For this review, use the dimensioned drawing (mm, ordinates from the lowest corner) and the shaded views. A direction names the side the tool comes from. Coordinates: 2 decimals unless noted, no trailing zeros. Write each loop counter-clockwise with the first axis right and the second up, starting at its lowest first coordinate (ties: lowest second). Pieces come first, ordered by that corner, then holes. Notation, with made-up numbers: M 27.25,49.25 L 69.25,49.25 A12 ccw 69.25,63.25 Z; hole C 1.25,35 d8. An arc over 180 degrees is marked long. One line per question, with ' | ' between items.
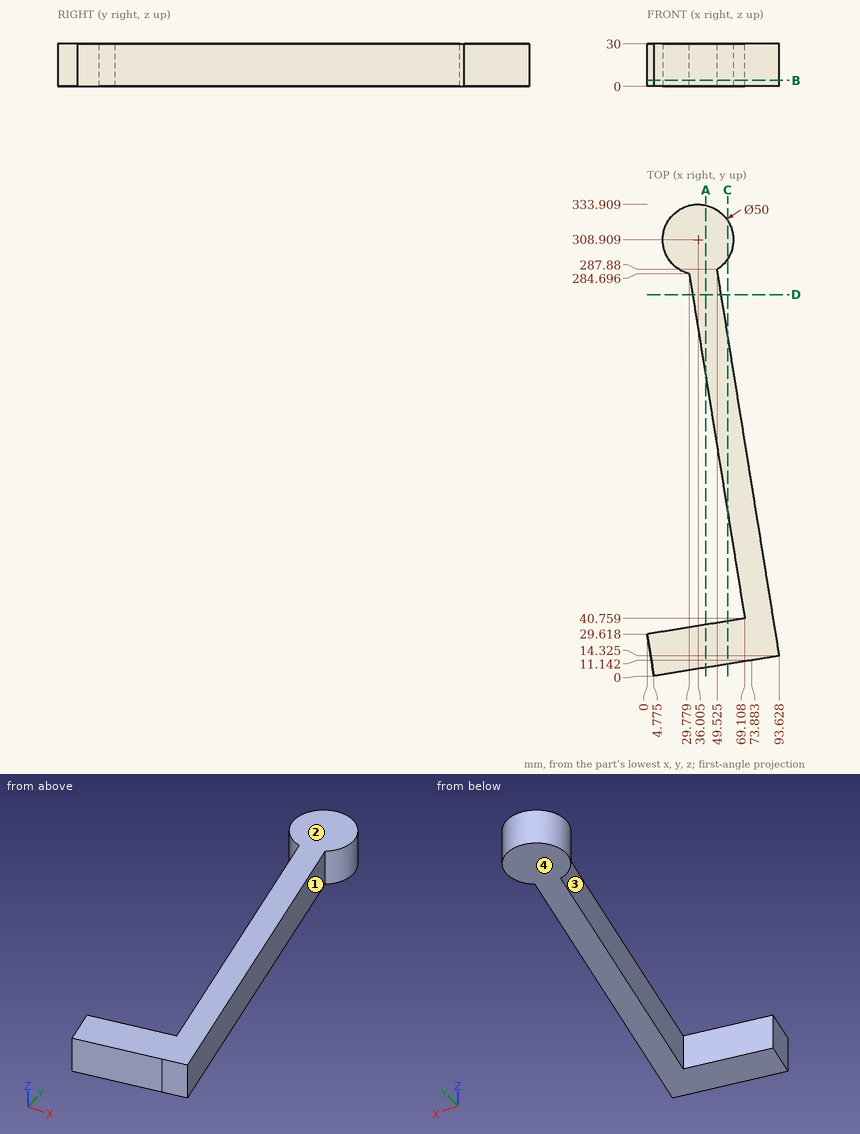
1) The part is to be moulded in two halves that separate along Y. For the marked faces 1 and 2, say which applies: +Y half, -Y half, draft (parallel to the pull), parting line (faces both ways), or undercut.
Responses:
face 1: undercut | face 2: draft
2) To check wall thickness, follow line 1 along Y through (x, z) = (21.5, 12.5) (1 decimal); line 2 along Y through (x, z) = (14.5, 23.25) (1 decimal); line 3 along X through (y, z) = (268, 25.25). State the ranges of each line that lie inside material, in increasing order. Write a range as [from, to].
Responses:
line 1: [2.7, 33.1], [288.5, 329.3] | line 2: [1.6, 32], [296.2, 321.7] | line 3: [32.47, 52.73]
3) Machinability: for the marked faces 3 and 4, which of the approach directions +Z, -Z, +X, -X, +Y, -Y give a long, thin tool a straight path to every point of the face, cutting with its end or side? Answer none if there is none.
Responses:
face 3: +Z, -Z, -X | face 4: -Z, +X, -X, +Y, -Y
4) Insertion check: pin 1 Ø1.5 at (y, z) = (66.5, 10.5) entering from +X; pin 2 Ø6 at (x, z) = (53, 21) entering from +Y (1 decimal); pin 3 Ø2 at (y, z) = (242.5, 13.5) entering from -X. Each pin has a flat end and moves straight along its axis. Give the tip position at first contact, or say it passes through.
Responses:
pin 1: x = 85.34 | pin 2: y = 329.6 | pin 3: x = 36.42
5) We need section D-D on y = 270. State the section outline as (x, z) points.
Responses:
outline: M 32.15,0 L 52.41,0 L 52.41,30 L 32.15,30 Z
6) We need section C-C on x = 57. State the section outline as (y, z) points.
Responses:
outline: M 8.42,0 L 38.81,0 L 38.81,30 L 8.42,30 Z; M 115.86,0 L 241.51,0 L 241.51,30 L 115.86,30 Z; M 295.34,0 L 322.48,0 L 322.48,30 L 295.34,30 Z
7) We need section B-B on z = 4.25. State the section outline as (x, y) points (1 decimal), then the cut area to 3 significant figures.
Responses:
outline: M 0,29.6 L 4.8,0 L 73.9,11.1 L 93.6,14.3 L 49.5,287.9 A25 ccw long 29.8,284.7 L 69.1,40.8 Z | area: 9,580 mm^2
8) We need section A-A on x = 41.5. State the section outline as (y, z) points, then the cut area to 3 significant figures.
Responses:
outline: M 5.92,0 L 36.31,0 L 36.31,30 L 5.92,30 Z; M 212,0 L 333.3,0 L 333.3,30 L 212,30 Z | area: 4,550 mm^2
